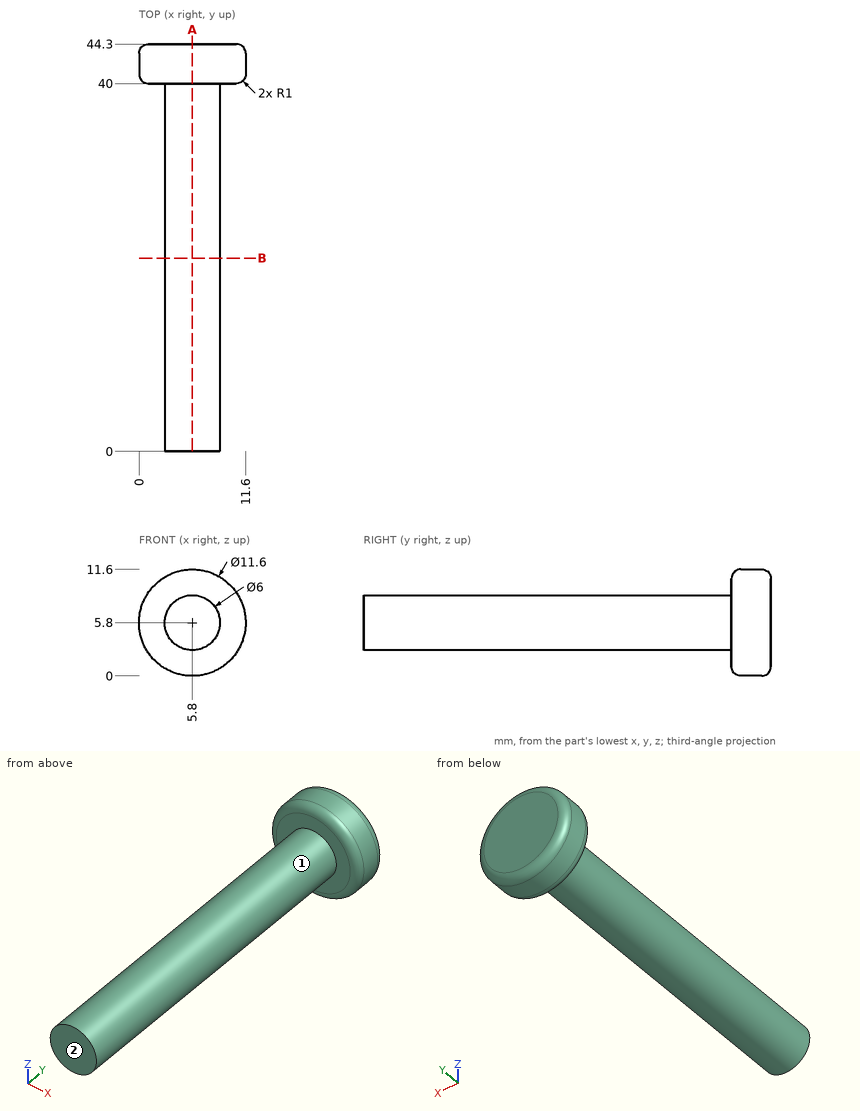
Input: dimensioned drawing with shaded views. Units: mm. Origin: part minimum x, y, z. A direction names the side the tool comes from. Give positions to 0.01 mm unless a question says otherwise; leave off trailing zeros. Loops run counter-clockwise (first coordinate to the right, second up) from the corner with the lowest first, then second, coordinate; pieces in that order, holes last. Notation, with made-up numbers: M 72,3 L 77,3 A21 cw 77,30 Z; hole C -27,-2.75 d2. An arc over 180 degrees is marked long. Put each result on its own line as item: value.
1) Cut plane A-A, the plane x = 5.8. Return the cut outline in (y, z).
Computed values:
outline: M 0,2.8 L 40,2.8 L 40,1 A1 ccw 41,0 L 43.3,0 A1 ccw 44.3,1 L 44.3,10.6 A1 ccw 43.3,11.6 L 41,11.6 A1 ccw 40,10.6 L 40,8.8 L 0,8.8 Z
2) Cut plane B-B, the plane y = 21. Return the cut outline in (x, z).
Computed values:
outline: C 5.8,5.8 d6
3) First-contact query: P1, Ø2, axis at y = 26, z = 5, coming from the +X side; P2, Ø5, axis at x = 5.5, y = 25, coming from the -Z side; P3, Ø6, axis at y = 9.5, z = 10, coming from the +X side. Flat tips, straight axial feed; report the tip coordinate or a pass-through.
Computed values:
P1: stops at x = 8.8
P2: stops at z = 2.8
P3: stops at x = 8.55
4) Reachability of the marked faces 1 and 2 from +Z, -Z, +X, -X, +Y, -Y: full face, straight path, thin tool, end or side. Return the list, or none.
Computed values:
face 1: -Y
face 2: +Z, -Z, +X, -X, -Y
5) Material intervals for L1, parallel to X at y = 9, z = 6; L2, parallel to Y at x = 3.5, z = 9; L3, parallel to X at y = 37, z = 7, sorted ascending. Write a range as from..to.
Computed values:
L1: x = 2.81..8.79
L2: y = 40..44.3
L3: x = 3.05..8.55
